Here's how the part is built. I have some questions about the finished solid (model axes, mm). A direction names the side the tool comes from. Round coordinates to 2 decimals unless told otherwise and drop trailing zeros. Write each loop counter-clockwise with the first axis right and the second up, starting at its lowest first coordinate (ties: lowest second). Pieces come first, ordered by that corner, then holes. Notation, with made-up numbers: (-29.5, 32) -> (21.5, 32) arc R12 cw to (21.5, 41) -> close; hole circle Ø2 at (29.5, 39.5). An arc over 180 degrees is marked (long way). Answer as CSV lines item,"result".
```python
from build123d import *

# Parameters (mm, degrees)
SKETCH1_W           = 3
SKETCH1_H           = 15
SKETCH1_W_2         = 80
SKETCH1_H_2         = 90
BOSS_EXTRUDE1_DEPTH = 3


with BuildPart() as part:
    # Sketch1 → Boss-Extrude1 (new body)
    with BuildSketch(Plane.XY):
        with Locations((-41.5, 0)):
            Rectangle(SKETCH1_W, SKETCH1_H)
        Rectangle(SKETCH1_W_2, SKETCH1_H_2)
        with Locations((41.5, 0)):
            Rectangle(SKETCH1_W, SKETCH1_H)
    extrude(amount=BOSS_EXTRUDE1_DEPTH)


solid = part.part
```
1. Suppose I cut it at B-B on y = 32.5. Please give me the cut outline in (x, z), and give its area (3 significant figures).
Numbers:
outline,"(-40, 0) -> (40, 0) -> (40, 3) -> (-40, 3) -> close"
area,"240 mm^2"
2. On a 3-axis mill with a long thin cutter (end or side, diameter ignored), from which of +Z, -Z, +X, -X, +Y, -Y can I reach the whole of each face in a straight line? I mean faces 1 (the face through (-40, -27, 1)), 2 (the face through (40, 26, 1)), 3 (the face through (41, -7.5, 1)), 4 (the face through (-42, 7.5, 1)). Say none if no direction works.
Numbers:
face 1,"+Z, -Z, -X, -Y"
face 2,"+Z, -Z, +X, +Y"
face 3,"+Z, -Z, +X, -Y"
face 4,"+Z, -Z, -X, +Y"
3. Suppose I cut it at A-A on z = 2.3. Please give me the cut outline in (x, y), and give its area (3 significant figures).
Numbers:
outline,"(-43, -7.5) -> (-40, -7.5) -> (-40, -45) -> (40, -45) -> (40, -7.5) -> (43, -7.5) -> (43, 7.5) -> (40, 7.5) -> (40, 45) -> (-40, 45) -> (-40, 7.5) -> (-43, 7.5) -> close"
area,"7,290 mm^2"
4. If I drill on line 1 (X direction, y = -10.5, z = 2.25), over which ranges is the centre line in solid material (lowest first)?
Numbers:
line 1,"x = -40 to 40"
5. For pin 1 Ø4 at (x, y) = (23, 30) entering from -Z; pin 2 Ø0.9 at (x, z) = (-41, 2) entering from +Y, each with a flat end and sliding along its axis, tell me the tip position at first contact or that it passes through.
Numbers:
pin 1,"stops at z = 0"
pin 2,"stops at y = 7.5"
